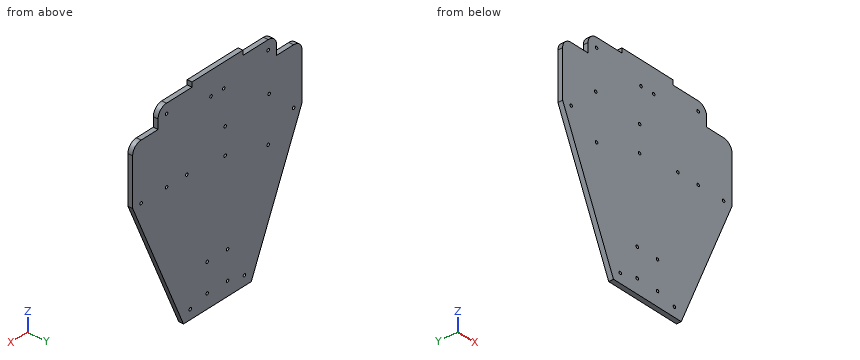
```python
from build123d import *

# Parameters (mm, degrees)
BOSS_EXTRUDE1_DEPTH = 5
SKETCH3_R           = 1.5
CUT_EXTRUDE2_DEPTH  = 6
SKETCH6_R           = 1.5
CUT_EXTRUDE4_DEPTH  = 6
SKETCH8_R           = 1.5
CUT_EXTRUDE5_DEPTH  = 10
SKETCH9_R           = 1.5
CUT_EXTRUDE6_DEPTH  = 10


with BuildPart() as part:
    # Sketch1 → Boss-Extrude1 (new body)
    with BuildSketch(Plane(origin=(0, 0, 0), x_dir=(1, 0, 0), z_dir=(0, 1, 0))):
        with BuildLine():
            Line((100, -40), (100, 10))
            Line((100, 10), (40, 150))
            Line((40, 150), (-40, 150))
            Line((-40, 150), (-100, 10))
            Line((-100, 10), (-100, -40))
            ThreePointArc((-100, -40), (-97.071067812, -47.071067812), (-90, -50))
            Line((-90, -50), (-70, -50))
            Line((-70, -50), (-70, -60))
            ThreePointArc((-70, -60), (-67.071067812, -67.071067812), (-60, -70))
            Line((-60, -70), (-30, -70))
            Line((-30, -70), (-30, -75))
            Line((-30, -75), (30, -75))
            Line((30, -75), (30, -70))
            Line((30, -70), (60, -70))
            ThreePointArc((60, -70), (67.071067812, -67.071067812), (70, -60))
            Line((70, -60), (70, -50))
            Line((70, -50), (90, -50))
            ThreePointArc((90, -50), (97.071067812, -47.071067812), (100, -40))
        make_face()
    extrude(amount=BOSS_EXTRUDE1_DEPTH)

    # Sketch3 → Cut-Extrude2 (cut, through all)
    with BuildSketch(Plane(origin=(0, 5, 0), x_dir=(1, 0, 0), z_dir=(0, 1, 0))):
        with Locations((-61.1, -17.8)):
            Circle(SKETCH3_R)
        with Locations((-9.2, -13.1)):
            Circle(SKETCH3_R)
        with Locations((-9.2, 14.8)):
            Circle(SKETCH3_R)
        with Locations((-60, 30)):
            Circle(SKETCH3_R)
    extrude(amount=-CUT_EXTRUDE2_DEPTH, mode=Mode.SUBTRACT)

    # Sketch6 → Cut-Extrude4 (cut, through all)
    with BuildSketch(Plane(origin=(0, 5, 0), x_dir=(1, 0, 0), z_dir=(0, 1, 0))):
        with Locations((12, 135)):
            Circle(SKETCH6_R)
        with Locations((-12, 135)):
            Circle(SKETCH6_R)
        with Locations((12, 105)):
            Circle(SKETCH6_R)
        with Locations((-12, 105)):
            Circle(SKETCH6_R)
    extrude(amount=-CUT_EXTRUDE4_DEPTH, mode=Mode.SUBTRACT)

    # Sketch8 → Cut-Extrude5 (cut)
    with BuildSketch(Plane(origin=(0, 5, 0), x_dir=(1, 0, 0), z_dir=(0, 1, 0))):
        with Locations((-90, 10)):
            Circle(SKETCH8_R)
        with Locations((-32, 140)):
            Circle(SKETCH8_R)
        with Locations((90, 10)):
            Circle(SKETCH8_R)
        with Locations((32, 140)):
            Circle(SKETCH8_R)
        with Locations((-60, -60)):
            Circle(SKETCH8_R)
        with Locations((60, -60)):
            Circle(SKETCH8_R)
        with Locations((-7.5, -50)):
            Circle(SKETCH8_R)
        with Locations((7.5, -50)):
            Circle(SKETCH8_R)
    extrude(amount=-CUT_EXTRUDE5_DEPTH, mode=Mode.SUBTRACT)

    # Sketch9 → Cut-Extrude6 (cut)
    with BuildSketch(Plane(origin=(0, 5, 0), x_dir=(1, 0, 0), z_dir=(0, 1, 0))):
        with Locations((60, 10)):
            Circle(SKETCH9_R)
        with Locations((36, 10)):
            Circle(SKETCH9_R)
    extrude(amount=-CUT_EXTRUDE6_DEPTH, mode=Mode.SUBTRACT)


solid = part.part
```
Can you work these out from the model? Positions are in its coordinate system, mm. Coordinates: 2 decimals unless noted, no trailing zeros. Order: outer loops, then holes, each group sorted by start corner. A loop starts at its lowest first (then second) coordinate and runs counter-clockwise, first axis right, second up.
1. If we section it at C-C (z = -61.5): Please give me the cut outline in (x, y).
2. If we section it at A-A (y = 1.5): Give the number of separate pieces and of enclosed holes in the cut face, then the cut area to 3 significant figures.
3. I need wall thicknesses on line 1 (Z direction, x = 12, y = 3.25); line 2 (X direction, y = 2.15, z = 13.1); line 3 (Z direction, x = 7.5, y = 3.2). Which ranges of each line are inside material? Lowest first, please.
4. If we section it at B-B (x = 82): Please give me the cut outline in (y, z).
5. I'm going to push flat-ended pins straight in: pin 1 (2.5 mm diameter, centred on x = -60, z = 60, fed in from -Y); pin 2 (2 mm diameter, centred on y = 4.5, z = -115.5, fed in from -X); pin 3 (2 mm diameter, centred on x = -54, y = 1, fed in from -Z); pin 4 (1.5 mm diameter, centred on x = 38.5, y = 1.5, fed in from +Z). Where does each tip first touch, or does it pass through?
Entries:
1. outline: (-77.93, 0) - (77.93, 0) - (77.93, 5) - (-77.93, 5) - close
2. separate pieces: 1
2. enclosed holes: 18
2. area: 34,500 mm2
3. line 1: z = -150 to -136.5, -133.5 to -106.5, -103.5 to 75
3. line 2: x = -100 to -10.7, -7.7 to 100
3. line 3: z = -150 to 48.5, 51.5 to 75
4. outline: (0, -52) - (5, -52) - (5, 50) - (0, 50) - close
5. pin 1: passes through
5. pin 2: stops at x = -55.21
5. pin 3: stops at z = -119.67
5. pin 4: stops at z = 70
